```python
from build123d import *

# Parameters (mm, degrees)
SALIENTE_EXTRUIR1_DEPTH  = 30.875
SALIENTE_EXTRUIR2_DEPTH  = 2
SALIENTE_EXTRUIR3_DEPTH  = 20
SALIENTE_EXTRUIR4_DEPTH  = 3
CROQUIS6_W               = 2
CROQUIS6_H               = 6
SALIENTE_EXTRUIR6_DEPTH  = 2.5
CORTAR_EXTRUIR1_REACH    = 63.75
SALIENTE_EXTRUIR7_DEPTH  = 4.2
SALIENTE_EXTRUIR9_DEPTH  = 1.35
CHAFL_N3_SIZE            = 0.75
REDONDEO1_R              = 0.5
CHAFL_N4_SIZE            = 1
CORTAR_EXTRUIR2_DEPTH    = 5.5
SALIENTE_EXTRUIR10_DEPTH = 10
CORTAR_EXTRUIR3_REACH    = 16.5
CROQUIS11_R              = 1.7
CROQUIS14_W              = 2.25
CROQUIS14_H              = 3.25
CORTAR_EXTRUIR6_DEPTH    = 11.500000101


with BuildPart() as part:
    # Croquis2 → Saliente-Extruir1 (new body, symmetric)
    with BuildSketch(Plane.YZ):
        with BuildLine():
            Line((0, -12.5), (0, -14.5))
            ThreePointArc((0, -14.5), (14.5, 0), (0, 14.5))
            Line((0, 14.5), (0, 12.5))
            ThreePointArc((0, 12.5), (12.5, 0), (0, -12.5))
        make_face()
    extrude(amount=SALIENTE_EXTRUIR1_DEPTH, both=True)

    # Croquis3 → Saliente-Extruir2 (add)
    with BuildSketch(Plane(origin=(-21.625, 0, 0), x_dir=(0, 0, -1), z_dir=(1, 0, 0))):
        with BuildLine():
            Line((-12.5, 0), (-3.75, 0))
            ThreePointArc((-3.75, 0), (0, 3.75), (3.75, 0))
            Line((3.75, 0), (12.5, 0))
            ThreePointArc((12.5, 0), (0, 12.5), (-12.5, 0))
        make_face()
    extrude(amount=-SALIENTE_EXTRUIR2_DEPTH)

    # Croquis4 → Saliente-Extruir3 (add)
    with BuildSketch(Plane(origin=(23.125, 0, 0), x_dir=(0, 0, -1), z_dir=(1, 0, 0))):
        with BuildLine():
            ThreePointArc((9.604686356, 8), (0, 12.5), (-9.604686356, 8))
            Line((-9.604686356, 8), (9.604686356, 8))
        make_face()
    extrude(amount=-SALIENTE_EXTRUIR3_DEPTH)

    # Croquis4_4 → Saliente-Extruir4 (add)
    with BuildSketch(Plane(origin=(23.125, 0, 0), x_dir=(0, 0, -1), z_dir=(1, 0, 0))):
        with BuildLine():
            ThreePointArc((9.604686356, 8), (0, 12.5), (-9.604686356, 8))
            Line((-9.604686356, 8), (9.604686356, 8))
        make_face()
        with BuildLine():
            ThreePointArc((-9.604686356, 8), (-10.908611376, 6.10345786), (-11.842719282, 4))
            Line((-11.842719282, 4), (-4.325, 4))
            Line((-4.325, 4), (4.325, 4))
            Line((4.325, 4), (11.842719282, 4))
            ThreePointArc((11.842719282, 4), (10.908611376, 6.10345786), (9.604686356, 8))
            Line((9.604686356, 8), (-9.604686356, 8))
        make_face()
    extrude(amount=SALIENTE_EXTRUIR4_DEPTH)

    # Croquis6 → Saliente-Extruir6 (add)
    with BuildSketch(Plane(origin=(0, 13.5, 0), x_dir=(-1, 0, 0), z_dir=(0, 1, 0))):
        with Locations((29.875, 0)):
            Rectangle(CROQUIS6_W, CROQUIS6_H)
    extrude(amount=-SALIENTE_EXTRUIR6_DEPTH)

    # Croquis7 → Cortar-Extruir1 (cut, up to next)
    with BuildSketch(Plane(origin=(-30.875, 0, 0), x_dir=(0, -1, 0), z_dir=(-1, 0, 0)), mode=Mode.PRIVATE) as cortar_extruir1_sk1:
        with BuildLine():
            ThreePointArc((-11, 3), (-11.401754251, 0), (-11, -3))
            Line((-11, -3), (-11, 3))
        make_face()
    cortar_extruir1_tool1 = extrude(cortar_extruir1_sk1.sketch, amount=-CORTAR_EXTRUIR1_REACH, mode=Mode.PRIVATE) & part.part
    add(cortar_extruir1_tool1.solids().sort_by_distance((-30.875, 11.160947, 0))[0], mode=Mode.SUBTRACT)

    # Croquis7_4 → Saliente-Extruir7 (add)
    with BuildSketch(Plane(origin=(-30.875, 0, 0), x_dir=(0, -1, 0), z_dir=(-1, 0, 0))):
        with BuildLine():
            ThreePointArc((-11, -3), (-11.401754251, 0), (-11, 3))
            Line((-11, 3), (-12.033432948, 3))
            ThreePointArc((-12.033432948, 3), (-12.401754251, 0), (-12.033432948, -3))
            Line((-12.033432948, -3), (-11, -3))
        make_face()
    extrude(amount=SALIENTE_EXTRUIR7_DEPTH)

    # Croquis8 → Saliente-Extruir9 (add)
    with BuildSketch(Plane(origin=(-35.075, 0, 0), x_dir=(0, -1, 0), z_dir=(-1, 0, 0))):
        with BuildLine():
            Line((-11, 3), (-13, 3))
            ThreePointArc((-13, 3), (-13.401754251, 0), (-13, -3))
            Line((-13, -3), (-11, -3))
            ThreePointArc((-11, -3), (-11.401754251, 0), (-11, 3))
        make_face()
    extrude(amount=-SALIENTE_EXTRUIR9_DEPTH)

    # Chafl_n3
    chafl_n3_edges = [part.edges().sort_by_distance(p)[0] for p in [
        (-35.075, 13.401754251, 0),
    ]]
    chamfer(chafl_n3_edges, length=CHAFL_N3_SIZE)

    # Redondeo1
    redondeo1_edges = [part.edges().sort_by_distance(p)[0] for p in [
        (-34.325, 13.401754251, 0),
    ]]
    fillet(redondeo1_edges, radius=REDONDEO1_R)

    # Chafl_n4
    chafl_n4_edges = [part.edges().sort_by_distance(p)[0] for p in [
        (-28.875, 12.5, 0),
    ]]
    chamfer(chafl_n4_edges, length=CHAFL_N4_SIZE)

    # Croquis9 → Cortar-Extruir2 (cut)
    with BuildSketch(Plane.YZ.offset(30.875)):
        with BuildLine():
            ThreePointArc((4, -11.842719282), (12.5, 0), (4, 11.842719282))
            Line((4, 11.842719282), (4, -11.842719282))
        make_face()
        with BuildLine():
            Line((0, 14.5), (0, 12.5))
            ThreePointArc((0, 12.5), (12.5, 0), (0, -12.5))
            Line((0, -12.5), (0, -14.5))
            ThreePointArc((0, -14.5), (14.5, 0), (0, 14.5))
        make_face()
    extrude(amount=-CORTAR_EXTRUIR2_DEPTH, mode=Mode.SUBTRACT)

    # Croquis10 → Saliente-Extruir10 (add)
    with BuildSketch(Plane.YZ.offset(25.375)):
        with BuildLine():
            Line((11.456439237, 5), (13.610657589, 5))
            ThreePointArc((13.610657589, 5), (14.5, 0), (13.610657589, -5))
            Line((13.610657589, -5), (11.456439237, -5))
            ThreePointArc((11.456439237, -5), (12.5, 0), (11.456439237, 5))
        make_face()
    extrude(amount=SALIENTE_EXTRUIR10_DEPTH)

    # Croquis11 → Cortar-Extruir3 (cut, up to next)
    with BuildSketch(Plane(origin=(0, 14.5, 0), x_dir=(-1, 0, 0), z_dir=(0, 1, 0)), mode=Mode.PRIVATE) as cortar_extruir3_sk1:
        with Locations((-30.375, 0)):
            Circle(CROQUIS11_R)
    cortar_extruir3_tool1 = extrude(cortar_extruir3_sk1.sketch, amount=-CORTAR_EXTRUIR3_REACH, mode=Mode.PRIVATE) & part.part
    add(cortar_extruir3_tool1.solids().sort_by_distance((30.375, 14.5, 0))[0], mode=Mode.SUBTRACT)

    # Croquis14 → Cortar-Extruir6 (cut, through all)
    with BuildSketch(Plane.XZ.offset(-4)):
        with Locations((24.25, 7.785)):
            Rectangle(CROQUIS14_W, CROQUIS14_H)
        with Locations((24.25, -7.785)):
            Rectangle(CROQUIS14_W, CROQUIS14_H)
    extrude(amount=-CORTAR_EXTRUIR6_DEPTH, mode=Mode.SUBTRACT)


solid = part.part
```
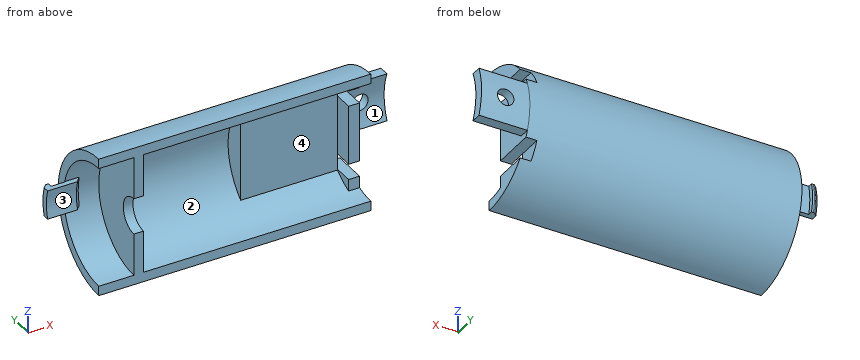
Part model, mm, in its own coordinate system. Face numbers are marked on the shaded views. A direction names the side the tool comes from. Give positions to 0.01 mm unless a question says otherwise; leave off trailing zeros. Write each loop counter-clockwise with the first axis right and the second up, starting at its lowest first coordinate (ties: lowest second). Pieces come first, ordered by that corner, then holes. Notation, with made-up numbers: (-37, 7) -> (18, 7) arc R25 cw to (18, 40) -> close; hole circle Ø2 at (32, 5). An arc over 180 degrees is marked (long way). Put each result on its own line as item: value. Start each with the question number.
Item 1: Wall check: L1, parallel to Z at x = -25, y = 5; L2, parallel to Z at x = -22, y = 2; L3, parallel to Y at x = 19, z = 0.25. Give the ranges that are in metal, low to high. Write a range as [from, to].
Item 2: Cut at B-B (y = 6.75). List the corners of the cut face in (x, z) (3 decimals).
Item 3: Pin check, flat tips, straight feed: pin 1 Ø5 at (x, y) = (-16, 7.5) entering from -Z; pin 2 Ø8 at (x, z) = (-2, 7) entering from +Y; pin 3 Ø2 at (x, y) = (-32.5, 11.5) entering from +Z; pin 4 Ø3 at (x, z) = (30.375, 0) entering from -Y. Stop position of each tip, or through.
Item 4: Cut at D-D (y = 9.5). List the corners of the cut face in (x, z) (3 decimals), then the cut area to 3 significant figures.
Item 5: Pull direction X, two halves, no side cores. Call the marked faces 3 and 4: pulls with the +X half, pulls with the -X half, needs draft (parallel to the pull), parting line crosses it, or undercut.
Item 6: Cut at A-A (x = 13.5). List the corners of the cut face in (y, z).
Item 7: Which spindle directions (+Z, -Z, +X, -X, +Y, -Y) get a long thin tool onto all of the face, cutting with end or side? Do the marked faces 1 and 2. Say none if no direction does.
Item 8: Cut at C-C (z = 10.25). List the corners of the cut face in (x, y) (3 decimals), then the cut area to 3 significant figures.
Answer list:
1. L1: z = [-13.61, -11.46], [11.46, 13.61]
1. L2: z = [-14.36, -3.17], [3.17, 14.36]
1. L3: y = [8, 14.5]
2. outline: (-30.875, -12.833) -> (25.375, -12.833) -> (25.375, -9.41) -> (23.125, -9.41) -> (23.125, -10.521) -> (-21.625, -10.521) -> (-21.625, 10.521) -> (23.125, 10.521) -> (23.125, 9.41) -> (25.375, 9.41) -> (25.375, 12.833) -> (-30.875, 12.833) -> (-30.875, 10.521) -> (-23.625, 10.521) -> (-23.625, -10.521) -> (-30.875, -10.521) -> close; (23.125, -6.16) -> (25.375, -6.16) -> (25.375, 6.16) -> (23.125, 6.16) -> close
3. pin 1: stops at z = -13.61
3. pin 2: stops at y = 14.19
3. pin 3: stops at z = 3
3. pin 4: passes through
4. outline: (-30.875, -10.954) -> (25.375, -10.954) -> (25.375, -9.41) -> (23.125, -9.41) -> (23.125, -6.16) -> (25.375, -6.16) -> (25.375, 6.16) -> (23.125, 6.16) -> (23.125, 9.41) -> (25.375, 9.41) -> (25.375, 10.954) -> (-30.875, 10.954) -> (-30.875, 8.124) -> (-23.625, 8.124) -> (-23.625, -8.124) -> (-30.875, -8.124) -> close; hole (-21.625, -8.124) -> (3.125, -8.124) -> (3.125, 8.124) -> (-21.625, 8.124) -> close
4. area: 698 mm2
5. face 3: needs draft
5. face 4: undercut
6. outline: (0, -14.5) arc R14.5 ccw to (0, 14.5) -> (0, 12.5) arc R12.5 cw to (8, 9.6) -> (8, -9.6) arc R12.5 cw to (0, -12.5) -> close
7. face 1: +X, -Y
7. face 2: -Y
8. outline: (-30.875, 7.155) -> (-23.625, 7.155) -> (-23.625, 0) -> (-21.625, 0) -> (-21.625, 7.155) -> (23.125, 7.155) -> (23.125, 4) -> (25.375, 4) -> (25.375, 10.256) -> (-30.875, 10.256) -> close
8. area: 196 mm2
